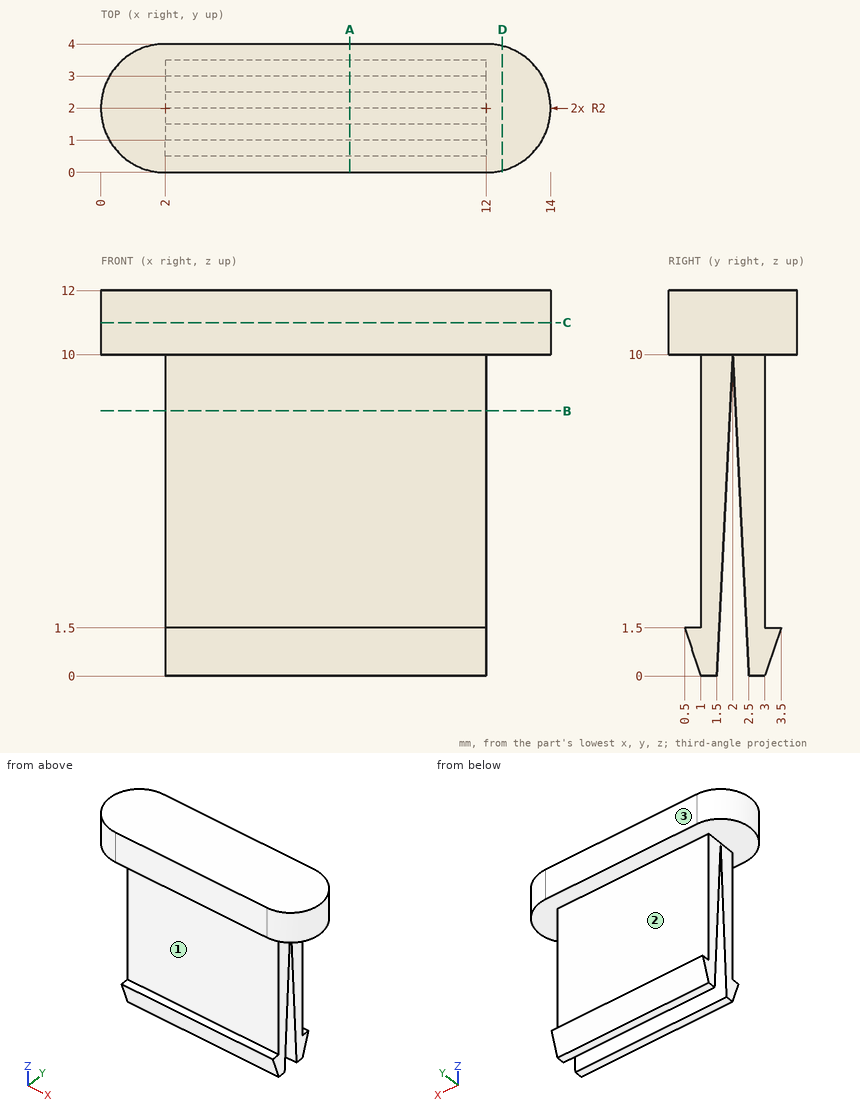
Study the drawing (mm; zero at the part's minimum x, y, z) and answer. A direction names the side the tool comes from. Coordinates: 2 decimals unless noted, no trailing zeros. Write each loop counter-clockwise with the first axis right and the second up, starting at its lowest first coordinate (ties: lowest second). Pieces come first, ordered by that corner, then holes.
Q1. Find the intervals of material crossed by line 1 along Z through (x, y) = (9.5, 0.2); line 2 along Y through (x, z) = (3, 6.5) (3 decimals); line 3 along Y through (x, z) = (7, 2), in increasing order.
Returned:
line 1: z = 10 to 12
line 2: y = 1 to 1.825, 2.175 to 3
line 3: y = 1 to 1.6, 2.4 to 3
Q2. Section A-A, the plane x = 7.75 is taken. Write down the section's boundary in (y, z).
Returned:
outline: (0, 10) - (1, 10) - (1, 1.5) - (0.5, 1.5) - (1, 0) - (1.5, 0) - (2, 10) - (2.5, 0) - (3, 0) - (3.5, 1.5) - (3, 1.5) - (3, 10) - (4, 10) - (4, 12) - (0, 12) - close
Q3. Section C-C, the plane z = 11 is taken. Write down the section's boundary in (x, y).
Returned:
outline: (2, 0) - (12, 0) arc R2 ccw to (12, 4) - (2, 4) arc R2 ccw to start
Q4. Which of the six approach directions +Z, -Z, +X, -X, +Y, -Y give full straight-line access (tool end or side, diameter ignored) to the marked faces 1, 2 and 3?
Returned:
face 1: +X, -X, -Y
face 2: +X, -X, +Y
face 3: +Z, -Z, +X, -X, +Y
Q5. Section B-B, the plane z = 8.25 is taken. Write down the section's boundary in (x, y).
Returned:
outline: (2, 1) - (12, 1) - (12, 1.91) - (2, 1.91) - close; (2, 2.09) - (12, 2.09) - (12, 3) - (2, 3) - close
Q6. Section D-D, the plane x = 12.5 is taken. Write down the section's boundary in (y, z), then the cut area to 3 significant figures.
Returned:
outline: (0.06, 10) - (3.94, 10) - (3.94, 12) - (0.06, 12) - close
area: 7.75 mm2
Q7. Given P1, Ø2.5, axis at x = 5.5, z = 6, coming from the -Y side; P2, Ø2.5, axis at x = 8, z = 6.5, coming from the +Y side; P3, Ø1, axis at y = 2.5, z = 7, coming from the -X side, each flat-ended and moving along its own axis, determine where each tip first touches the part or whether it passes through.
Returned:
P1: stops at y = 1
P2: stops at y = 3
P3: stops at x = 2
